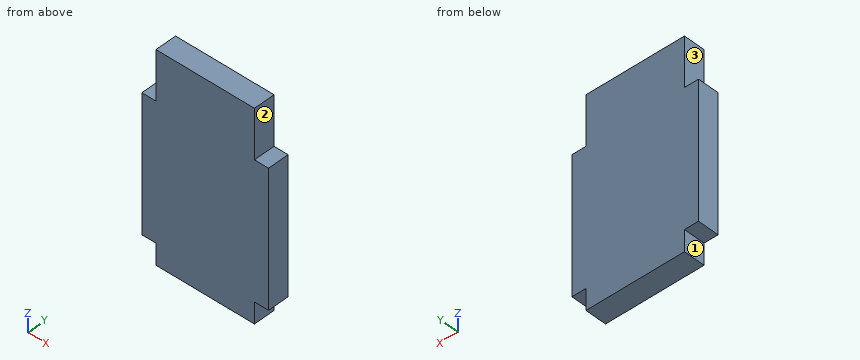
```python
from build123d import *

# Parameters (mm, degrees)
EXTRUDE_1_DEPTH = 3
SKETCH_3_W      = 14
SKETCH_3_H      = 3
EXTRUDE_2_DEPTH = 4


with BuildPart() as part:
    # Эскиз1 → Бобышка-Вытянуть1 (new body)
    with BuildSketch(Plane(origin=(0, 0, 0), x_dir=(1, 0, 0), z_dir=(0, 1, 0))):
        Polygon((-9, -10.434482278), (-9, 8.865517722), (-7, 8.865517722), (-7, 11.865517722), (7, 11.865517722), (7, 8.865517722), (9, 8.865517722), (9, -10.434482278), (7, -10.434482278), (7, -13.434482278), (-7, -13.434482278), (-7, -10.434482278), align=None)
    extrude(amount=EXTRUDE_1_DEPTH)

    # Эскиз3 → Бобышка-Вытянуть2 (add)
    with BuildSketch(Plane.XY.offset(13.434482278)):
        with Locations((0, 1.5)):
            Rectangle(SKETCH_3_W, SKETCH_3_H)
    extrude(amount=EXTRUDE_2_DEPTH)


solid = part.part
```
CAD build for the part. Positions are in the model's coordinates, mm. Face numbers are marked on the shaded views. A direction names the side the tool comes from. Round coordinates to 2 decimals unless told otherwise and drop trailing zeros. Order: outer loops, then holes, each group sorted by start corner. A loop starts at its lowest first (then second) coordinate and runs counter-clockwise, first axis right, second up. Notation, with made-up numbers: (32.25, 86) - (40.25, 86) arc R13 ccw to (40.25, 103) - close; hole circle Ø6 at (-12.75, 29.25). An arc over 180 degrees is marked (long way). Answer in a Markdown table with one row per item. Add a question column.
(1) 3-axis set-ups, long thin cutter, end or side, ignore diameter. For the marked faces 1, 2 and 3: which of +Z, -Z, +X, -X, +Y, -Y reach the whole face in a straight line?
(2) Drop flat-ended pins along their axis: pin 1 Ø1.5 at (y, z) = (1.5, -11) entering from +X; pin 2 Ø0.9 at (y, z) = (1.5, 14.5) entering from -X; pin 3 Ø1 at (x, y) = (8.5, 1) entering from +Z. Give the stop position or say it passes through.
(3) Band-saw the part on A-A on y = 1.65. List the corners of the cut face in (x, z), and give its area (3 significant figures).
(4) Band-saw the part on C-C on x = -7.5. List the corners of the cut face in (y, z), and give its area (3 significant figures).
(5) Band-saw the part on B-B on z = 15. List the corners of the cut face in (x, y).
(6) Probe L1, parallel to Z at x = 8, y = 2.65; L2, parallel to X at y = 1.15, z = 12.25. List the from-to ranges inside material, lowest first. Write a range as [from, to].
Data:
| question | item | result |
|---|---|---|
| 1 | face 1 | -Z, -X, +Y, -Y |
| 1 | face 2 | +Z, +X, +Y, -Y |
| 1 | face 3 | +Z, -X, +Y, -Y |
| 2 | pin 1 | stops at x = 7 |
| 2 | pin 2 | stops at x = -7 |
| 2 | pin 3 | stops at z = 10.43 |
| 3 | outline | (-9, -8.87) - (-7, -8.87) - (-7, -11.87) - (7, -11.87) - (7, -8.87) - (9, -8.87) - (9, 10.43) - (7, 10.43) - (7, 17.43) - (-7, 17.43) - (-7, 10.43) - (-9, 10.43) - close |
| 3 | area | 487 mm^2 |
| 4 | outline | (0, -8.87) - (3, -8.87) - (3, 10.43) - (0, 10.43) - close |
| 4 | area | 57.9 mm^2 |
| 5 | outline | (-7, 0) - (7, 0) - (7, 3) - (-7, 3) - close |
| 6 | L1 | z = [-8.87, 10.43] |
| 6 | L2 | x = [-7, 7] |
